Verification items for this drawing (mm, ordinates from the low corner). Round coordinates to 2 decimals unless told otherwise and drop trailing zeros. Order: outer loops, then holes, each group sorted by start corner. A loop starts at its lowest first (then second) coordinate and runs counter-clockwise, first axis right, second up. Notation, with made-up numbers: (-6, -6) - (46, -6) arc R17 ccw to (46, 24) - close; hole circle Ø9 at (1.25, 46.25). An arc over 180 degrees is marked (long way). Return JSON: item names as keys, results as strings. Group by question number.
Q1. Material ranges on line 1 along Y through (x, z) = (101, 89.5); line 2 along X through (y, z) = (107, 14); line 3 along Z through (x, y) = (651, 700.5), recorded low to high.
Q2. Gauge pin test, flat end, axial feed: pin 1 Ø8 at (x, y) = (349.5, 294) entering from +Z. Record the tip position at first contact, or that the pin passes through.
Q3. Sectioned sample at B-B, the plane x = 410.5. Record the cut outline in (y, z).
Q4. Sectioned sample at C-C, the plane y = 291.5. Record the cut outline in (x, z).
Q5. Draft check along Y on the marked faces 1, 2, 3 and 4. Enter one of: pulls with the +Y half, pulls with the -Y half, needs draft (parallel to the pull), parting line crosses it, or undercut.
Q6. Sectioned sample at A-A, the plane z = 91. Record the cut outline in (x, y), then the cut area to 3 significant figures.
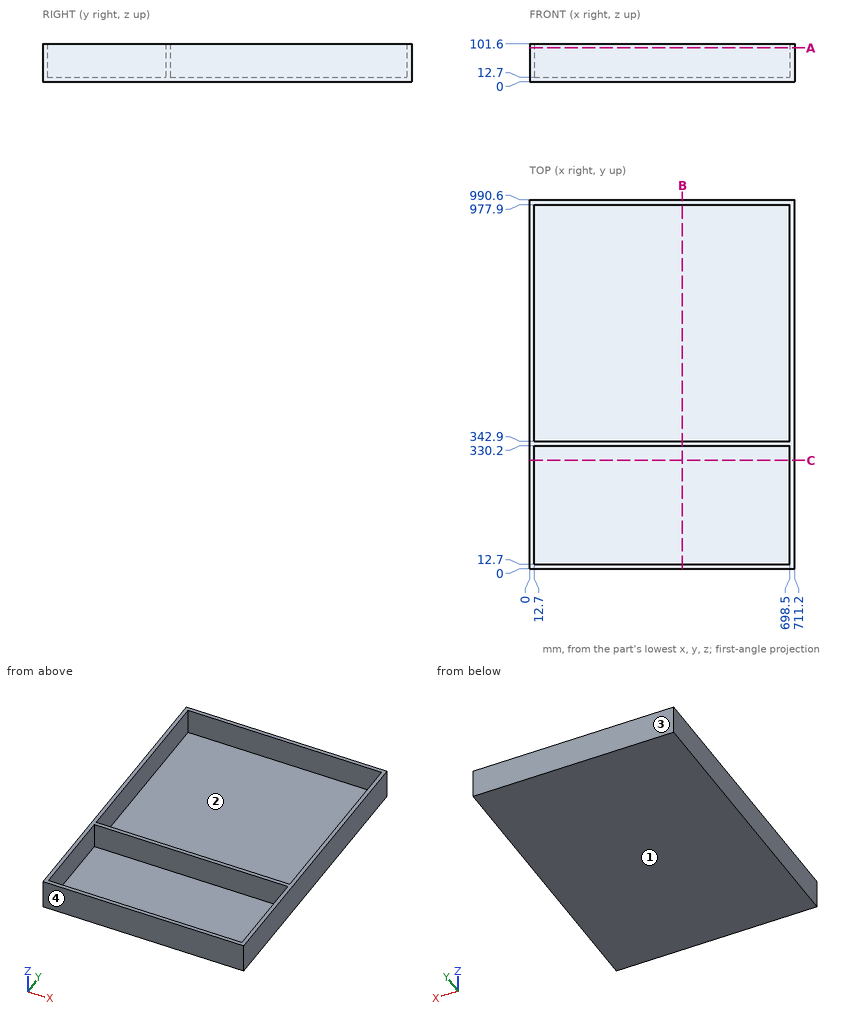
Reply:
{
 "1": {"line 1": "0 to 12.7, 330.2 to 342.9, 977.9 to 990.6", "line 2": "0 to 12.7, 698.5 to 711.2", "line 3": "0 to 12.7"},
 "2": {"pin 1": "z = 12.7"},
 "3": {"outline": "(0, 0) - (990.6, 0) - (990.6, 101.6) - (977.9, 101.6) - (977.9, 12.7) - (342.9, 12.7) - (342.9, 101.6) - (330.2, 101.6) - (330.2, 12.7) - (12.7, 12.7) - (12.7, 101.6) - (0, 101.6) - close"},
 "4": {"outline": "(0, 0) - (711.2, 0) - (711.2, 101.6) - (698.5, 101.6) - (698.5, 12.7) - (12.7, 12.7) - (12.7, 101.6) - (0, 101.6) - close"},
 "5": {"face 1": "needs draft", "face 2": "undercut", "face 3": "pulls with the +Y half", "face 4": "pulls with the -Y half"},
 "6": {"outline": "(0, 0) - (711.2, 0) - (711.2, 990.6) - (0, 990.6) - close; hole (12.7, 12.7) - (698.5, 12.7) - (698.5, 330.2) - (12.7, 330.2) - close; hole (12.7, 342.9) - (698.5, 342.9) - (698.5, 977.9) - (12.7, 977.9) - close", "area": "51,300 mm^2"}
}
